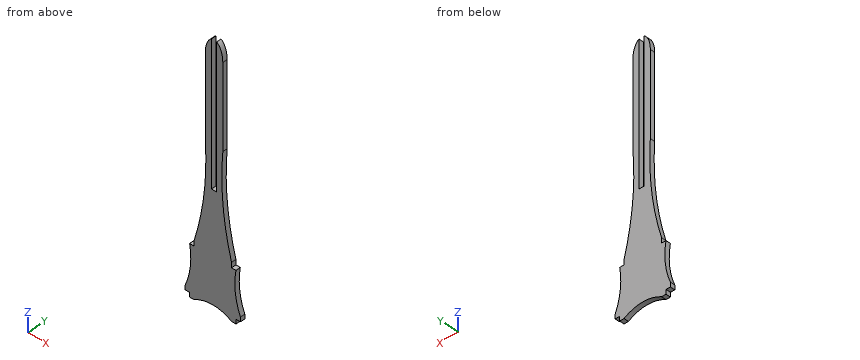
from build123d import *

# Parameters (mm, degrees)
F1_DEPTH = 3.175


# Not quite as in the source:
# - a length typed as a fraction of an inch, garbled in the dataset ("3 / 203.2 mm" for 3/8 in), is restored


with BuildPart() as f1:
    # F0 (on Front) → F1 (new body)
    with BuildSketch(Plane.XZ):
        with BuildLine():
            add(Edge.make_bspline(
                [(-1.75, 126.1528220874), (-5.9, 123.6896499738), (-5.9, 115.3852411336)],
                knots=[3.4427337756, 3.4427337756, 3.4427337756, 4.7123889804, 4.7123889804, 4.7123889804], degree=2, weights=[1, 0.8051739469, 1]))
            Line((-5.9, 115.3852411336), (-1.75, 115.3852411336))
            Line((-1.75, 115.3852411336), (-1.75, 126.1528220874))
        make_face()
        with BuildLine():
            add(Edge.make_bspline(
                [(-5.9, 115.3852411336), (-5.9, 107.0808322935), (-1.75, 104.6176601799)],
                knots=[4.7123889804, 4.7123889804, 4.7123889804, 5.9820441852, 5.9820441852, 5.9820441852], degree=2, weights=[1, 0.8051739469, 1]))
            Line((-5.9, 115.3852411336), (-5.9, 79.8345449512))
            Line((-5.9, 79.8345449512), (-5.9, 58.9576361328))
            ThreePointArc((-5.9, 58.9576361328), (-6.7793812573, 25.2130721087), (-13.4661033603, -7.8740350493))
            Line((-13.4661033603, -7.8740350493), (11.7832735849, -7.8740350493))
            ThreePointArc((11.7832735849, -7.8740350493), (5.9964918029, 25.2913389557), (5.9, 58.9576361328))
            Line((5.9, 58.9576361328), (5.9, 79.8345449512))
            Line((5.9, 79.8345449512), (5.9, 115.3852411336))
            add(Edge.make_bspline(
                [(1.75, 104.6176601799), (5.9, 107.0808322935), (5.9, 115.3852411336)],
                knots=[0.301141122, 0.301141122, 0.301141122, 1.5707963268, 1.5707963268, 1.5707963268], degree=2, weights=[1, 0.8051739469, 1]))
            Line((1.75, 104.6176601799), (1.75, 31.1528220874))
            Line((1.75, 31.1528220874), (-1.75, 31.1528220874))
            Line((-1.75, 31.1528220874), (-1.75, 104.6176601799))
        make_face()
        with BuildLine():
            Line((-1.75, 115.3852411336), (-5.9, 115.3852411336))
            add(Edge.make_bspline(
                [(-5.9, 115.3852411336), (-5.9, 107.0808322935), (-1.75, 104.6176601799)],
                knots=[4.7123889804, 4.7123889804, 4.7123889804, 5.9820441852, 5.9820441852, 5.9820441852], degree=2, weights=[1, 0.8051739469, 1]))
            Line((-1.75, 104.6176601799), (-1.75, 115.3852411336))
        make_face()
        with BuildLine():
            Line((1.75, 126.1528220874), (1.75, 115.3852411336))
            Line((1.75, 115.3852411336), (5.9, 115.3852411336))
            add(Edge.make_bspline(
                [(5.9, 115.3852411336), (5.9, 123.6896499738), (1.75, 126.1528220874)],
                knots=[1.5707963268, 1.5707963268, 1.5707963268, 2.8404515316, 2.8404515316, 2.8404515316], degree=2, weights=[1, 0.8051739469, 1]))
        make_face()
        with BuildLine():
            Line((5.9, 115.3852411336), (1.75, 115.3852411336))
            Line((1.75, 115.3852411336), (1.75, 104.6176601799))
            add(Edge.make_bspline(
                [(1.75, 104.6176601799), (5.9, 107.0808322935), (5.9, 115.3852411336)],
                knots=[0.301141122, 0.301141122, 0.301141122, 1.5707963268, 1.5707963268, 1.5707963268], degree=2, weights=[1, 0.8051739469, 1]))
        make_face()
        with BuildLine():
            Line((11.7832735849, -7.8740350493), (-13.4661033603, -7.8740350493))
            Line((-13.4661033603, -7.8740350493), (-13.4661033603, -11.3740350493))
            Line((-13.4661033603, -11.3740350493), (-16.4661033603, -11.3740350493))
            ThreePointArc((-16.4661033603, -11.3740350493), (-15.9973063906, -25.5681128526), (-19.4661033603, -39.3397889622))
            Line((-19.4661033603, -39.3397889622), (-19.4661033603, -42.3397889622))
            Line((-19.4661033603, -42.3397889622), (-16.5214760231, -42.3397889622))
            Line((-16.5214760231, -42.3397889622), (-16.5214760231, -45.3397889622))
            Line((-16.5214760231, -45.3397889622), (-13.5214760231, -45.3397889622))
            ThreePointArc((-13.5214760231, -45.3397889622), (-0.8691012191, -41.7016149524), (11.7832735849, -45.3397889622))
            Line((11.7832735849, -45.3397889622), (14.7832735849, -45.3397889622))
            Line((14.7832735849, -45.3397889622), (14.7832735849, -42.3397889622))
            Line((14.7832735849, -42.3397889622), (17.7832735849, -42.3397889622))
            Line((17.7832735849, -42.3397889622), (17.7832735849, -39.3397889622))
            ThreePointArc((17.7832735849, -39.3397889622), (14.302318759, -25.5694170752), (14.7832735849, -11.3740350493))
            Line((14.7832735849, -11.3740350493), (11.7832735849, -11.3740350493))
            Line((11.7832735849, -11.3740350493), (11.7832735849, -7.8740350493))
        make_face()
    extrude(amount=F1_DEPTH)


solid = f1.part
Check sheet for the modelled part. Datum: model origin and axes. Units: mm. Round coordinates to 2 decimals unless told otherwise and drop trailing zeros. Order: outer loops, then holes, each group sorted by start corner. A loop starts at its lowest first (then second) coordinate and runs counter-clockwise, first axis right, second up.
(1) Go/stop test with flat-tipped pins: P1, Ø0.9, axis at x = 17, y = -1, coming from the -Z side; P2, Ø1, axis at y = -1.5, z = 98, coming from the +X side; P3, Ø0.9, axis at x = -15, y = -1.5, coming from the +Z side. Record where each tip stops, or that it passes through.
(2) Cross-section at A-A, the plane z = 71. Enter the section's corners in (x, y) (3 decimals), and give its area (3 significant figures).
(3) Scan lines: probe 1 along X at (y, z) = (-0.7, 91.5); probe 2 along Z at (x, y) = (-0.5, -0.3); probe 3 along Z at (x, y) = (13.5, -2.45). Record each from-to range of solid material in increasing order.
(4) Cross-section at C-C, the plane z = -9.5. Enter the section's corners in (x, y) (3 decimals).
(5) Cross-section at D-D, the plane x = -8. Enter the section's corners in (y, z) (3 decimals).
Check sheet entries:
1. P1: stops at z = -42.34
1. P2: stops at x = 5.9
1. P3: stops at z = -11.37
2. outline: (-5.9, -3.175) - (-1.75, -3.175) - (-1.75, 0) - (-5.9, 0) - close; (1.75, -3.175) - (5.9, -3.175) - (5.9, 0) - (1.75, 0) - close
2. area: 26.4 mm2
3. probe 1: x = -5.9 to -1.75, 1.75 to 5.9
3. probe 2: z = -41.7 to 31.15
3. probe 3: z = -45.34 to -11.37
4. outline: (-13.466, -3.175) - (11.783, -3.175) - (11.783, 0) - (-13.466, 0) - close
5. outline: (-3.175, -42.794) - (0, -42.794) - (0, 16.283) - (-3.175, 16.283) - close
